The drawing under review shows one solid part. Ordinate dimensions are in mm from its lowest x, y, z. Give positions to 0.01 mm unless a question says otherwise; leave off trailing zeros. Loops run counter-clockwise (first coordinate to the right, second up) from the corner with the lowest first, then second, coordinate; pieces in that order, holes last. Notation, with made-up numbers: (-39.5, -36.5) -> (3.5, -36.5) arc R28 ccw to (3.5, -5.5) -> close; hole circle Ø5 at (64, 61.25). An arc over 180 degrees is marked (long way). Answer in a Markdown table with one row per item. Add a question column.
(1) For line 1 (Z direction, x = 826.5, y = 214.5); line 2 (Y direction, x = 277.5, z = 918), list the stretches that pass through material, from the lowest coordinate up.
(2) For pin 1 (22 mm diameter, centred on x = 983.5, y = 244, fed in from -Z); pin 2 (8 mm diameter, centred on x = 660.5, y = 395.5, fed in from -Z); pin 3 (15 mm diameter, centred on x = 966.5, z = 539, fed in from -Y), all flat-tipped, find the tip position at first contact; note any pin that passes through.
(3) Draft analysis for pull direction X (two halves, no side actions). For the marked faces 1 and 2, state which applies: +X half, -X half, draft (parallel to the pull), parting line (faces both ways), or undercut.
(4) Consider section C-C on x = 210. Write out the cut boundary in (y, z).
(5) Consider section A-A on z = 435.5. Write out the cut boundary in (x, y), then the cut area to 3 significant figures.
(6) Consider section B-B on y = 241. Write out the cut boundary in (x, z).
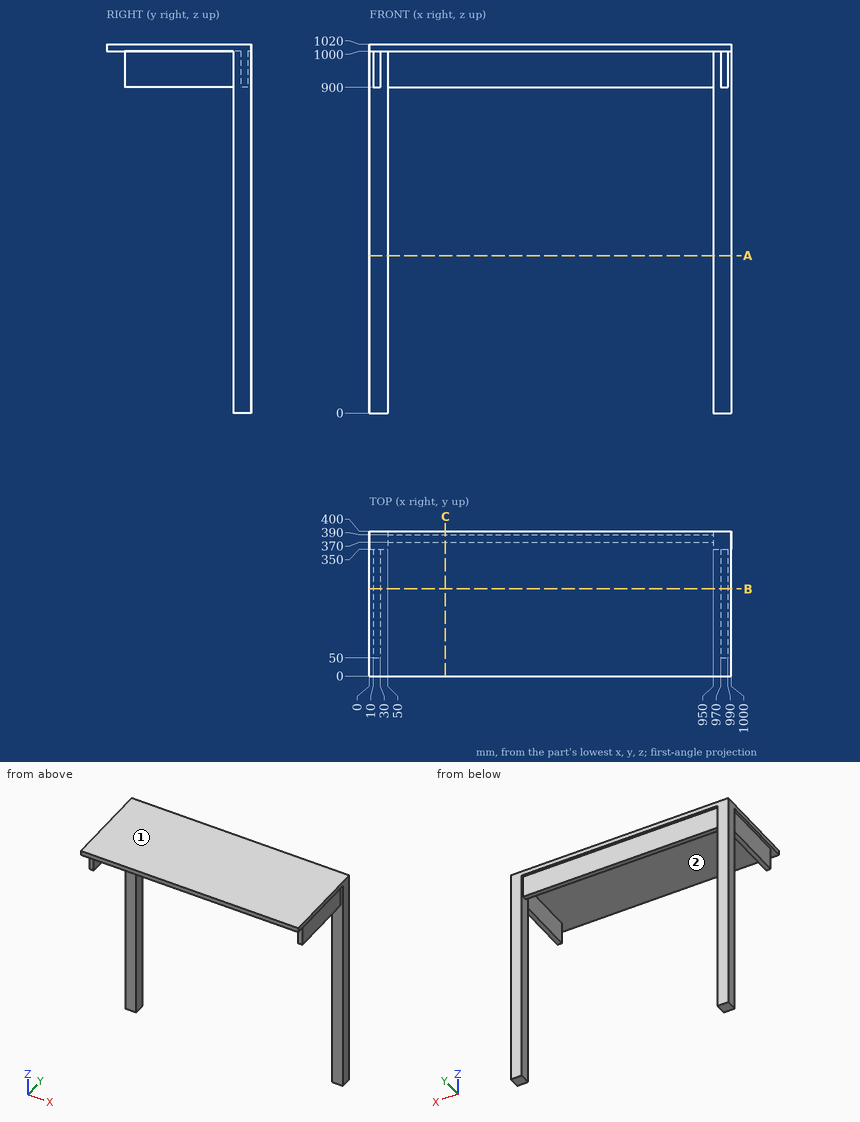
Values follow:
| question | item | result |
|---|---|---|
| 1 | line 1 | 1000 to 1020 |
| 1 | line 2 | 370 to 390 |
| 2 | pin 1 | z = 900 |
| 2 | pin 2 | z = 1000 |
| 2 | pin 3 | y = 350 |
| 3 | face 1 | draft |
| 3 | face 2 | undercut |
| 4 | outline | (0, 1000) -> (370, 1000) -> (370, 900) -> (390, 900) -> (390, 1000) -> (400, 1000) -> (400, 1020) -> (0, 1020) -> close |
| 5 | outline | (0, 350) -> (50, 350) -> (50, 400) -> (0, 400) -> close; (950, 350) -> (1000, 350) -> (1000, 400) -> (950, 400) -> close |
| 5 | area | 5,000 mm2 |
| 6 | outline | (0, 1000) -> (10, 1000) -> (10, 900) -> (30, 900) -> (30, 1000) -> (970, 1000) -> (970, 900) -> (990, 900) -> (990, 1000) -> (1000, 1000) -> (1000, 1020) -> (0, 1020) -> close |
